Work out the finished part from the listing and answer in its coordinate system (mm). Face numbers are marked on the shaded views. A direction names the side the tool comes from. Coordinates: 2 decimals unless noted, no trailing zeros. Write each loop counter-clockwise with the first axis right and the second up, starting at its lowest first coordinate (ties: lowest second). Pieces come first, ordered by that corner, then holes. Notation, with made-up numbers: (23, -8) - (79, -8) arc R22 cw to (79, 16) - close; hole circle Ø9 at (55, 7). An arc over 180 degrees is marked (long way). Use one line per item in the form item = value. Start each with the question number.
Item 1: Determine the mould class of the marked faces 1, 2 and 3 for opening direction Y: released by +Y, released by -Y, zero draft, split by the parting line, or undercut.
Item 2: Consider probe 1 along Y at (x, z) = (8.55, 0.35); probe 2 along Z at (x, y) = (6.75, -1.5); probe 3 along Y at (x, z) = (4.55, 0.8). Determine where each line is inside the solid, lowest interval first.
Item 3: A cutting plane is placed at D-D (y = -3). Write down the section's boundary in (x, z), then the cut area to 3 significant figures.
Item 4: Given pin 1 (3 mm diameter, centred on x = 9, y = 0.5, fed in from +Z); pin 2 (2.5 mm diameter, centred on x = 0.5, y = 0, fed in from -Z); pin 3 (3 mm diameter, centred on x = 0, y = 0, fed in from +Z), each flat-ended and moving along its own axis, determine where each tip first touches the part or whether it passes through.
Item 5: A cutting plane is placed at B-B (x = 12.55). Write down the section's boundary in (y, z).
Item 6: A cutting plane is placed at A-A (z = 0.25). Write down the section's boundary in (x, y), then the cut area to 3 significant figures.
Item 7: A cutting plane is placed at C-C (x = 10.55). Write down the section's boundary in (y, z).
Item 8: For the marked faces 4, 5 and 6, determine the directions among +Z, -Z, +X, -X, +Y, -Y from which every point of the face is accessible in a straight line to the end or side of a thin tool.
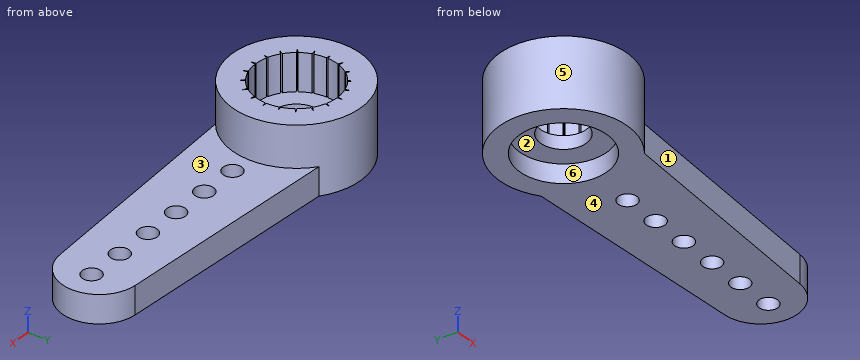
from build123d import *
from build123d.topology import SkipClean

# Parameters (mm, degrees)
EXTRUDE_1_DEPTH          = 1.5
SKETCH_2_R               = 3.45
EXTRUDE_2_DEPTH          = 2.2
SKETCH_4_R               = 1.225
CUT_EXTRUDE_2_DEPTH      = 17.780718101
SKETCH_3_R               = 2.175
CUT_EXTRUDE_1_DEPTH      = 2
CUT_EXTRUDE_3_DEPTH      = 2
PATTERN_CIRCULAR_1_COUNT = 20
SKETCH_6_R               = 2.35
CUT_EXTRUDE_4_DEPTH      = 1
SKETCH_7_R               = 0.5
CUT_EXTRUDE_5_DEPTH      = 17.514917499
CUT_EXTRUDE_6_DEPTH      = 17.780718101


with BuildPart() as part:
    # 草图1 → 凸台-拉伸1 (new body)
    with BuildSketch(Plane.XY):
        with BuildLine():
            Line((-14.124971514, 1.996091711), (-2.083266666, 2.75))
            ThreePointArc((-2.083266666, 2.75), (0, 3.45), (2.083266666, 2.75))
            Line((2.083266666, 2.75), (14.124971514, 1.996091711))
            ThreePointArc((14.124971514, 1.996091711), (16, 0), (14.124971514, -1.996091711))
            Line((14.124971514, -1.996091711), (2.083266666, -2.75))
            ThreePointArc((2.083266666, -2.75), (0, -3.45), (-2.083266666, -2.75))
            Line((-2.083266666, -2.75), (-14.124971514, -1.996091711))
            ThreePointArc((-14.124971514, -1.996091711), (-16, 0), (-14.124971514, 1.996091711))
        make_face()
    extrude(amount=EXTRUDE_1_DEPTH)

    # 草图2 → 凸台-拉伸2 (add)
    with SkipClean():  # the faces are left unmerged after this step: merging them gives an invalid solid
        with BuildSketch(Plane.XY.offset(1.5)):
            with Locations(Location((0, 0, 0), (0, 0, 127.145804172))):
                Circle(SKETCH_2_R)
        extrude(amount=EXTRUDE_2_DEPTH)

    # 草图4 → 切除-拉伸2 (cut, through all)
    with SkipClean():  # the faces are left unmerged after this step: merging them gives an invalid solid
        with BuildSketch(Plane(origin=(0, 0, 0), x_dir=(-1, 0, 0), z_dir=(0, 0, -1))):
            Circle(SKETCH_4_R)
        extrude(amount=-CUT_EXTRUDE_2_DEPTH, mode=Mode.SUBTRACT)

    # 草图3 → 切除-拉伸1 (cut)
    with SkipClean():  # the faces are left unmerged after this step: merging them gives an invalid solid
        with BuildSketch(Plane.XY.offset(3.7)):
            Circle(SKETCH_3_R)
        extrude(amount=-CUT_EXTRUDE_1_DEPTH, mode=Mode.SUBTRACT)

    # 草图5 → 切除-拉伸3 (cut)
    with SkipClean():  # the faces are left unmerged after this step: merging them gives an invalid solid
        with BuildSketch(Plane.XY.offset(3.7)):
            Polygon((2.425, 0), (1.700332145, 0.114776113), (1.700332145, -0.114776113), align=None)
        cut_extrude_3 = extrude(amount=-CUT_EXTRUDE_3_DEPTH, mode=Mode.SUBTRACT)

    # 阵列(圆周)1: 切除-拉伸3 ×20 about axis
    with SkipClean():  # the faces are left unmerged after this step: merging them gives an invalid solid
        pattern_circular_1_axis = Axis((0, 0, 0), (0, 0, 1))
        for i in range(1, PATTERN_CIRCULAR_1_COUNT):
            add(cut_extrude_3.rotate(pattern_circular_1_axis, i * 360 / PATTERN_CIRCULAR_1_COUNT), mode=Mode.SUBTRACT)

    # 草图6 → 切除-拉伸4 (cut)
    with SkipClean():  # the faces are left unmerged after this step: merging them gives an invalid solid
        with BuildSketch(Plane(origin=(0, 0, 0), x_dir=(-1, 0, 0), z_dir=(0, 0, -1))):
            Circle(SKETCH_6_R)
        extrude(amount=-CUT_EXTRUDE_4_DEPTH, mode=Mode.SUBTRACT)

    # 草图7 → 切除-拉伸5 (cut, through all)
    with SkipClean():  # the faces are left unmerged after this step: merging them gives an invalid solid
        with BuildSketch(Plane.XY.offset(1.5)):
            with Locations((-4.55, 0)):
                Circle(SKETCH_7_R)
            with Locations((-6.55, 0)):
                Circle(SKETCH_7_R)
            with Locations((-8.55, 0)):
                Circle(SKETCH_7_R)
            with Locations((-10.55, 0)):
                Circle(SKETCH_7_R)
            with Locations((-12.55, 0)):
                Circle(SKETCH_7_R)
            with Locations((-14.55, 0)):
                Circle(SKETCH_7_R)
        cut_extrude_5 = extrude(amount=-CUT_EXTRUDE_5_DEPTH, mode=Mode.SUBTRACT)

    # 镜向1: 切除-拉伸5 across plane
    with SkipClean():  # the faces are left unmerged after this step: merging them gives an invalid solid
        add(cut_extrude_5.mirror(Plane(origin=(0, 0, 0), x_dir=(0, 0, 1), z_dir=(1, 0, 0))), mode=Mode.SUBTRACT)

    # 草图8 → 切除-拉伸6 (cut, through all)
    with SkipClean():  # the faces are left unmerged after this step: merging them gives an invalid solid
        with BuildSketch(Plane.XY.offset(3.7)):
            with BuildLine():
                Line((-2.083266666, 2.75), (-16, 2.75))
                Line((-16, 2.75), (-16, -2.75))
                Line((-16, -2.75), (-2.083266666, -2.75))
                ThreePointArc((-2.083266666, -2.75), (-3.45, 0), (-2.083266666, 2.75))
            make_face()
        extrude(amount=-CUT_EXTRUDE_6_DEPTH, mode=Mode.SUBTRACT)


solid = part.part
Answer:
q1.face_1 = released by -Y
q1.face_2 = undercut
q1.face_3 = zero draft
q2.probe_1 = -2.35 to -0.5, 0.5 to 2.35
q2.probe_2 = 0 to 1.5
q2.probe_3 = -2.6 to -0.5, 0.5 to 2.6
q3.outline = (-1.7, 0) - (1.7, 0) - (1.7, 3.7) - (-1.7, 3.7) - close
q3.area = 12.6 mm²
q4.pin_1 = 1.5
q4.pin_2 = 1
q4.pin_3 = 1.7
q5.outline = (-2.09, 0) - (-0.5, 0) - (-0.5, 1.5) - (-2.09, 1.5) - close; (0.5, 0) - (2.09, 0) - (2.09, 1.5) - (0.5, 1.5) - close
q6.outline = (2.08, -2.75) - (14.12, -2) arc R2 ccw to (14.12, 2) - (2.08, 2.75) arc R3.45 ccw (long way) to start; hole circle Ø4.7 at (0, 0); hole circle Ø1 at (4.55, 0); hole circle Ø1 at (6.55, 0); hole circle Ø1 at (8.55, 0); hole circle Ø1 at (10.55, 0); hole circle Ø1 at (12.55, 0); hole circle Ø1 at (14.55, 0)
q6.area = 73.0 mm²
q7.outline = (-2.22, 0) - (-0.5, 0) - (-0.5, 1.5) - (-2.22, 1.5) - close; (0.5, 0) - (2.22, 0) - (2.22, 1.5) - (0.5, 1.5) - close
q8.face_4 = -Z, +X, -X, +Y, -Y
q8.face_5 = +Z
q8.face_6 = -Z
